The model under review builds one solid part; all positions refer to its coordinate system, in mm. Face numbers are marked on the shaded views. A direction names the side the tool comes from. Coordinates: 2 decimals unless noted, no trailing zeros. Order: outer loops, then holes, each group sorted by start corner. A loop starts at its lowest first (then second) coordinate and runs counter-clockwise, first axis right, second up. Notation, with made-up numbers: (58, 38) -> (103, 38) arc R13 cw to (103, 56) -> close; hole circle Ø6 at (-9.75, 70.5). An arc over 180 degrees is marked (long way). Use one line per item in the form item = value.
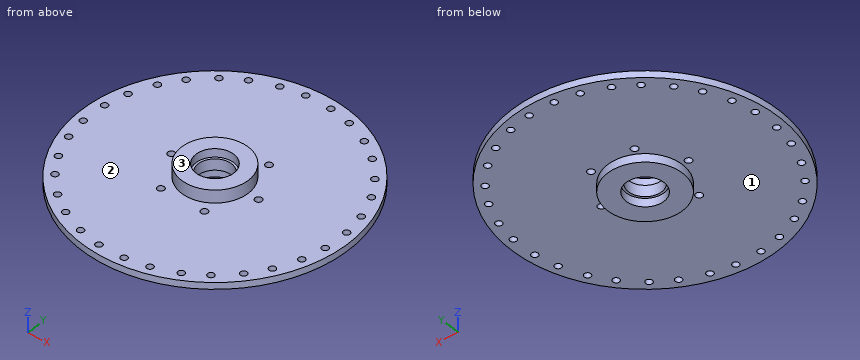
from build123d import *

# Parameters (mm, degrees)
SCHIZZO1_R                   = 240
SCHIZZO1_R_2                 = 6.25
ESTRUSIONE_ESTRUSIONE1_DEPTH = 12
SCHIZZO2_R                   = 60
ESTRUSIONE_ESTRUSIONE2_DEPTH = 23
SCHIZZO3_R                   = 67.5
ESTRUSIONE_ESTRUSIONE3_DEPTH = 15
SCHIZZO4_R                   = 34
TAGLIO_ESTRUSIONE1_DEPTH     = 15
SCHIZZO5_R                   = 30
TAGLIO_ESTRUSIONE2_DEPTH     = 20
TAGLIO_ESTRUSIONE3_START     = -15
SCHIZZO6_R                   = 34
TAGLIO_ESTRUSIONE3_DEPTH     = 15
SCHIZZO7_R                   = 6
TAGLIO_ESTRUSIONE4_DEPTH     = 12
RIPETIZIONECIRCOLARE1_COUNT  = 16


with BuildPart() as part:
    # Schizzo1 → Estrusione-Estrusione1 (new body)
    with BuildSketch(Plane.XY):
        Circle(SCHIZZO1_R)
        with Locations((-40, -69.282032303)):
            Circle(SCHIZZO1_R_2, mode=Mode.SUBTRACT)
        with Locations((40, -69.282032303)):
            Circle(SCHIZZO1_R_2, mode=Mode.SUBTRACT)
        with Locations((80, 0)):
            Circle(SCHIZZO1_R_2, mode=Mode.SUBTRACT)
        with Locations((40, 69.282032303)):
            Circle(SCHIZZO1_R_2, mode=Mode.SUBTRACT)
        with Locations((-40, 69.282032303)):
            Circle(SCHIZZO1_R_2, mode=Mode.SUBTRACT)
        with Locations((-80, 0)):
            Circle(SCHIZZO1_R_2, mode=Mode.SUBTRACT)
    extrude(amount=ESTRUSIONE_ESTRUSIONE1_DEPTH)

    # Schizzo2 → Estrusione-Estrusione2 (add)
    with BuildSketch(Plane.XY.offset(12)):
        Circle(SCHIZZO2_R)
    extrude(amount=ESTRUSIONE_ESTRUSIONE2_DEPTH)

    # Schizzo3 → Estrusione-Estrusione3 (add)
    with BuildSketch(Plane(origin=(0, 0, 0), x_dir=(-1, 0, 0), z_dir=(0, 0, -1))):
        with Locations(Location((0, 0, 0), (0, 0, 180))):
            Circle(SCHIZZO3_R)
    extrude(amount=ESTRUSIONE_ESTRUSIONE3_DEPTH)

    # Schizzo4 → Taglio-Estrusione1 (cut)
    with BuildSketch(Plane.XY.offset(35)):
        Circle(SCHIZZO4_R)
    extrude(amount=-TAGLIO_ESTRUSIONE1_DEPTH, mode=Mode.SUBTRACT)

    # Schizzo5 → Taglio-Estrusione2 (cut)
    with BuildSketch(Plane.XY.offset(20)):
        Circle(SCHIZZO5_R)
    extrude(amount=-TAGLIO_ESTRUSIONE2_DEPTH, mode=Mode.SUBTRACT)

    # Schizzo6 → Taglio-Estrusione3 (cut)
    with BuildSketch(Plane(origin=(0, 0, -15), x_dir=(-1, 0, 0), z_dir=(0, 0, -1)).offset(TAGLIO_ESTRUSIONE3_START)):
        with Locations(Location((0, 0, 0), (0, 0, 180))):
            Circle(SCHIZZO6_R)
    extrude(amount=TAGLIO_ESTRUSIONE3_DEPTH, mode=Mode.SUBTRACT)

    # Schizzo7 → Taglio-Estrusione4 (cut)
    with BuildSketch(Plane.XY.offset(12)):
        with Locations((-222, 23)):
            Circle(SCHIZZO7_R)
        with Locations((-222, -23)):
            Circle(SCHIZZO7_R)
    taglio_estrusione4 = extrude(amount=-TAGLIO_ESTRUSIONE4_DEPTH, mode=Mode.SUBTRACT)

    # RipetizioneCircolare1: Taglio-Estrusione4 ×16 about axis
    ripetizionecircolare1_axis = Axis((0, 0, 0), (0, 0, 1))
    for i in range(1, RIPETIZIONECIRCOLARE1_COUNT):
        add(taglio_estrusione4.rotate(ripetizionecircolare1_axis, i * 360 / RIPETIZIONECIRCOLARE1_COUNT), mode=Mode.SUBTRACT)


solid = part.part
Item 1: To check wall thickness, follow L1, parallel to X at y = 222, z = 8; L2, parallel to Z at x = 169.5, y = 74; L3, parallel to Y at x = 217, z = 11. State the ranges of each line that lie inside material, in increasing order. Write a range as from..to.
Results found:
L1 = -91.19..-29, -17..17, 29..91.19
L2 = 0..12
L3 = -102.52..-68.85, -58.57..-26.32, -19.68..19.68, 26.32..58.57, 68.85..102.52
Item 2: Clearance check with flat-ended pins moving along their axes: pin 1 (6 mm diameter, centred on y = 59, z = -3.5, fed in from -X); pin 2 (8 mm diameter, centred on x = -104.5, y = -55.5, fed in from +Z); pin 3 (1.5 mm diameter, centred on y = -127.5, z = 2.5, fed in from -X). State where each tip first meets the part, or that it passes through.
Results found:
pin_1 = -37.69
pin_2 = 12
pin_3 = -203.8
Item 3: Tool access review of the marked faces 1, 2 and 3: name each direction out of +Z, -Z, +X, -X, +Y, -Y from which nothing blocks a thin tool from reaching the whole face with its end or side.
Results found:
face_1 = -Z
face_2 = +Z
face_3 = +Z, +X, -X, +Y, -Y
Item 4: We need section D-D (y = -92). Write out the cut boundary in (x, z), plus the area to 3 significant figures.
Results found:
outline = (-221.67, 0) -> (221.67, 0) -> (221.67, 12) -> (-221.67, 12) -> close
area = 5,320 mm²
Item 5: We need section C-C (x = 23). State how many separate pieces and enclosed holes the cut face has, plus the area to 3 significant figures.
Results found:
separate_pieces = 4
enclosed_holes = 0
area = 7,630 mm²
Item 6: We need section A-A (x = 80). Write out the cut boundary in (y, z).
Results found:
outline = (-226.27, 0) -> (-6.25, 0) -> (-6.25, 12) -> (-226.27, 12) -> close; (6.25, 0) -> (226.27, 0) -> (226.27, 12) -> (6.25, 12) -> close
Item 7: We need section B-B (z = -5.5). Write out the cut boundary in (x, y).
Results found:
outline = circle Ø135 at (0, 0); hole circle Ø68 at (0, 0)
